Build history of the part. All positions in model axes, mm. A direction names the side the tool comes from. Give positions to 0.01 mm unless a question says otherwise; leave off trailing zeros. Loops run counter-clockwise (first coordinate to the right, second up) from the corner with the lowest first, then second, coordinate; pieces in that order, holes last.
1) Wall check: line 1 (X direction, y = 7.5, z = 0); line 2 (Z direction, x = -11.75, y = 4); line 3 (X direction, y = 1.3, z = 0). Give the ranges that are in metal, low to high.
2) Flat gauge pins, fed straight in: P1, Ø4, axis at x = 9.5, y = 13.5, coming from the +Z side; P2, Ø5, axis at x = -4, z = -1, coming from the +Y side; P3, Ø4, axis at x = 7, y = 12, coming from the -Z side; P4, Ø1.5, axis at y = 8.5, z = -3.5, coming from the +X side. Where does each tip first touch, or does it go through?
3) Band-saw the part on D-D on z = -5.5. List the corners of the cut face in (x, y), then the cut area to 3 significant figures.
4) 3-axis set-ups, long thin cutter, end or side, ignore diameter. For faces 1 (the flat face through (-15, 2, 5)), 2 (the flat face through (13, 2, 3)), 3 (the flat face through (-7, 5, 2)), 4 (the flat face through (-13, 2, 3)): which of +Z, -Z, +X, -X, +Y, -Y reach the whole face in a straight line?
5) Band-saw the part on C-C on y = 2. List the corners of the cut face in (x, z), then the cut area to 3 significant figures.
6) Band-saw the part on B-B on z = 0. List the corners of the cut face in (x, y), then the cut area to 3 significant figures.
7) Two-plate mould, pull along Z, no slides. Class faces 5 (the flat face through (13, 2, -3)), 6 (the flat face through (-15, 2, -5)), 7 (the flat face through (0, 2, 7.5)): +Z half, -Z half, draft (parallel to the pull), parting line (faces both ways), or undercut.
8) Band-saw the part on A-A on x = 0. List the corners of the cut face in (y, z).
```python
from build123d import *

# Parameters (mm, degrees)
EXTRUDE_1_DEPTH     = 5
SKETCH_3_R          = 7
SKETCH_3_R_2        = 4.5
EXTRUDE_2_DEPTH     = 11
SKETCH_3_3_R        = 4.5
CUT_EXTRUDE_1_DEPTH = 21.05617112


with BuildPart() as part:
    # Sketch 2 → Extrude 1 (new body)
    with BuildSketch(Plane(origin=(0, 0, 0), x_dir=(1, 0, 0), z_dir=(0, 1, 0))):
        with BuildLine():
            Line((-15, -7.5), (15, -7.5))
            Line((15, -7.5), (15, -3))
            Line((15, -3), (11, -3))
            ThreePointArc((11, -3), (8, 0), (11, 3))
            Line((11, 3), (15, 3))
            Line((15, 3), (15, 7.5))
            Line((15, 7.5), (-15, 7.5))
            Line((-15, 7.5), (-15, 3))
            Line((-15, 3), (-11, 3))
            ThreePointArc((-11, 3), (-8, 0), (-11, -3))
            Line((-11, -3), (-15, -3))
            Line((-15, -3), (-15, -7.5))
        make_face()
    extrude(amount=EXTRUDE_1_DEPTH)

    # Sketch 3 → Extrude 2 (add)
    with BuildSketch(Plane(origin=(0, 5, 0), x_dir=(1, 0, 0), z_dir=(0, 1, 0))):
        with Locations(Location((0, 0, 0), (0, 0, 270))):
            Circle(SKETCH_3_R)
        with Locations(Location((0, 0, 0), (0, 0, 270))):
            Circle(SKETCH_3_R_2, mode=Mode.SUBTRACT)
    extrude(amount=EXTRUDE_2_DEPTH)

    # Sketch 3_3 → Cut-Extrude 1 (cut, through all)
    with BuildSketch(Plane(origin=(0, 5, 0), x_dir=(1, 0, 0), z_dir=(0, 1, 0))):
        with Locations(Location((0, 0, 0), (0, 0, 270))):
            Circle(SKETCH_3_3_R)
    extrude(amount=-CUT_EXTRUDE_1_DEPTH, mode=Mode.SUBTRACT)


solid = part.part
```
Findings below:
1. line 1: x = -7 to -4.5, 4.5 to 7
1. line 2: z = -7.5 to -3, 3 to 7.5
1. line 3: x = -8 to -4.5, 4.5 to 8
2. P1: passes through
2. P2: stops at y = 16
2. P3: stops at z = -4.9
2. P4: stops at x = 6.44
3. outline: (-15, 0) - (15, 0) - (15, 5) - (4.33, 5) - (4.33, 16) - (-4.33, 16) - (-4.33, 5) - (-15, 5) - close
3. area: 245 mm2
4. face 1: +Z, -Z, -X, +Y, -Y
4. face 2: +X, +Y, -Y
4. face 3: +Y
4. face 4: -X, +Y, -Y
5. outline: (-15, -7.5) - (15, -7.5) - (15, -3) - (11, -3) arc R3 cw to (11, 3) - (15, 3) - (15, 7.5) - (-15, 7.5) - (-15, 3) - (-11, 3) arc R3 cw to (-11, -3) - (-15, -3) - close; hole circle Ø9 at (0, 0)
5. area: 310 mm2
6. outline: (-8, 0) - (-4.5, 0) - (-4.5, 16) - (-7, 16) - (-7, 5) - (-8, 5) - close; (4.5, 0) - (8, 0) - (8, 5) - (7, 5) - (7, 16) - (4.5, 16) - close
6. area: 90.0 mm2
7. face 5: undercut
7. face 6: draft
7. face 7: +Z half
8. outline: (0, -7.5) - (5, -7.5) - (5, -7) - (16, -7) - (16, -4.5) - (0, -4.5) - close; (0, 4.5) - (16, 4.5) - (16, 7) - (5, 7) - (5, 7.5) - (0, 7.5) - close
